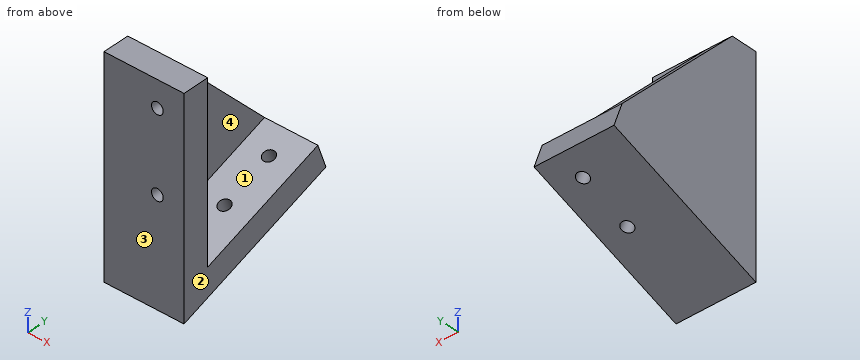
```python
from build123d import *

# Parameters (mm, degrees)
SKETCH1_W           = 15
SKETCH1_H           = 30
BOSS_EXTRUDE1_DEPTH = 40
CUT_EXTRUDE1_DEPTH  = 40
BOSS_EXTRUDE2_DEPTH = 10
CUT_EXTRUDE2_DEPTH  = 10
CUT_EXTRUDE3_DEPTH  = 10
SKETCH7_R           = 1.1
CUT_EXTRUDE4_DEPTH  = 10
SKETCH8_R           = 1.1
CUT_EXTRUDE5_DEPTH  = 10


with BuildPart() as part:
    # Sketch1 → Boss-Extrude1 (new body)
    with BuildSketch(Plane.XY):
        with Locations((7.5, 15)):
            Rectangle(SKETCH1_W, SKETCH1_H)
    extrude(amount=BOSS_EXTRUDE1_DEPTH)

    # Sketch2 → Cut-Extrude1 (cut)
    with BuildSketch(Plane(origin=(15, 0, 0), x_dir=(0, 0, -1), z_dir=(1, 0, 0))):
        Polygon((0, 0), (-10.919107028, 30), (0, 30), align=None)
    extrude(amount=-CUT_EXTRUDE1_DEPTH, mode=Mode.SUBTRACT)

    # Sketch3 → Boss-Extrude2 (add)
    with BuildSketch(Plane(origin=(15, 0, 0), x_dir=(0, 0, -1), z_dir=(1, 0, 0))):
        Polygon((-10.919107028, 30), (-15.617570132, 28.289899283), (-7.140740034, 5), (-40, 5), (-40, 0), (0, 0), align=None)
    extrude(amount=BOSS_EXTRUDE2_DEPTH)

    # Sketch5 → Cut-Extrude2 (cut)
    with BuildSketch(Plane.ZY):
        Polygon((10.919107028, 30), (40, 30), (40, 0), (0, 0), align=None)
    extrude(amount=-CUT_EXTRUDE2_DEPTH, mode=Mode.SUBTRACT)

    # Sketch6 → Cut-Extrude3 (cut)
    with BuildSketch(Plane(origin=(15, 0, 0), x_dir=(0, 0, -1), z_dir=(1, 0, 0))):
        Polygon((-15.617570132, 28.289899283), (-40, 5), (-40, 30), (-10.919107028, 30), align=None)
    extrude(amount=-CUT_EXTRUDE3_DEPTH, mode=Mode.SUBTRACT)

    # Sketch7 → Cut-Extrude4 (cut)
    with BuildSketch(Plane.XZ):
        with Locations(Location((20, 35, 0), (0, 0, 270))):
            Circle(SKETCH7_R)
        with Locations(Location((20, 20, 0), (0, 0, 270))):
            Circle(SKETCH7_R)
    extrude(amount=-CUT_EXTRUDE4_DEPTH, mode=Mode.SUBTRACT)

    # Sketch8 → Cut-Extrude5 (cut)
    with BuildSketch(Plane(origin=(0, 0, 0), x_dir=(-1, 0, 0), z_dir=(0, 0.342020143325663, -0.9396926207859105))):
        with Locations(Location((-20, 26.925333174, 0), (0, 0, 90))):
            Circle(SKETCH8_R)
        with Locations(Location((-20, 16.925333174, 0), (0, 0, 90))):
            Circle(SKETCH8_R)
    extrude(amount=-CUT_EXTRUDE5_DEPTH, mode=Mode.SUBTRACT)


solid = part.part
```
Check sheet for the modelled part. Datum: model origin and axes. Units: mm. Face numbers are marked on the shaded views. Round coordinates to 2 decimals unless told otherwise and drop trailing zeros. Order: outer loops, then holes, each group sorted by start corner. A loop starts at its lowest first (then second) coordinate and runs counter-clockwise, first axis right, second up. Notation, with made-up numbers: (75.5, -22.75) - (107.5, -22.75) arc R23 ccw to (107.5, -9.75) - close; hole circle Ø2 at (86.25, 34.5). An arc over 180 degrees is marked (long way). Write item = value, one per line.
Q1. Section check C-C (x = 11.5). Record the boundary of the cut face in (y, z).
Computed:
outline = (0, 0) - (30, 10.92) - (28.29, 15.62) - (5, 40) - (0, 40) - close
Q2. Go/stop test with flat-tipped pins: pin 1 (4 mm diameter, centred on y = 9, z = 19, fed in from +X); pin 2 (2 mm diameter, centred on x = 20, z = 20, fed in from +Y); pin 3 (5 mm diameter, centred on x = 22, z = 30, fed in from +Y). Record where each tip stops, or that it passes through.
Computed:
pin_1 = 15
pin_2 = through
pin_3 = 5
Q3. Section check D-D (z = 20). Record the boundary of the cut face in (x, y), and give its area (3 significant figures).
Computed:
outline = (10, 0) - (18.9, 0) - (18.9, 5) - (15, 5) - (15, 24.1) - (10, 24.1) - close; (21.1, 0) - (25, 0) - (25, 5) - (21.1, 5) - close
area = 160 mm^2
Q4. Section check A-A (z = 35). Record the boundary of the cut face in (x, y), and give its area (3 significant figures).
Computed:
outline = (10, 0) - (18.9, 0) - (18.9, 5) - (15, 5) - (15, 9.78) - (10, 9.78) - close; (21.1, 0) - (25, 0) - (25, 5) - (21.1, 5) - close
area = 87.9 mm^2
Q5. Thickness scan on line 1 along X through (y, z) = (1.9, 35); line 2 along Y through (x, z) = (23.5, 29.5); line 3 along X through (y, z) = (7.5, 15.5). Record the ranges inside material, lowest first.
Computed:
line_1 = 10 to 18.9, 21.1 to 25
line_2 = 0 to 5
line_3 = 10 to 15
Q6. Section check B-B (x = 20). Record the boundary of the cut face in (y, z).
Computed:
outline = (0, 0) - (14.87, 5.41) - (13.16, 10.11) - (5, 7.14) - (5, 18.9) - (0, 18.9) - close; (0, 21.1) - (5, 21.1) - (5, 33.9) - (0, 33.9) - close; (0, 36.1) - (5, 36.1) - (5, 40) - (0, 40) - close; (15.23, 10.86) - (16.94, 6.17) - (24.27, 8.83) - (22.56, 13.53) - close; (24.63, 14.28) - (26.34, 9.59) - (30, 10.92) - (28.29, 15.62) - close
Q7. Draft check along Y on the marked faces 1, 2, 3 and 4. Enter one of: pulls with the +Y half, pulls with the -Y half, needs draft (parallel to the pull), parting line crosses it, or undercut.
Computed:
face_1 = undercut
face_2 = needs draft
face_3 = pulls with the -Y half
face_4 = undercut
